For this review, take the finished solid that the model builds, in its own axes (mm). Face numbers are marked on the shaded views. A direction names the side the tool comes from. Round coordinates to 2 decimals unless told otherwise and drop trailing zeros. Write each loop counter-clockwise with the first axis right and the second up, starting at its lowest first coordinate (ties: lowest second). Pieces come first, ordered by that corner, then holes. Notation, with made-up numbers: (48, 11) -> (78, 11) arc R8 cw to (78, 24) -> close; hole circle Ø10 at (72, 12.5). An arc over 180 degrees is marked (long way). Answer as CSV lines item,"result". Start each with the question number.
Item 1: Take a section at A-A on y = 11.7. Count the separate pieces of the cut face and the enclosed holes in it, then the cut area to 3 significant figures.
Item 2: Machinability: for the marked faces 1, 2 and 3, which of the approach directions +Z, -Z, +X, -X, +Y, -Y give a long, thin tool a straight path to every point of the face, cutting with its end or side? Answer none if there is none.
Item 3: Wall thickness on probe 1 along X at (y, z) = (11, 8); probe 2 along Z at (x, y) = (13.5, 3.5); probe 3 along Y at (x, z) = (8.75, 7): over which ranges is each line inside the solid? List them lowest first. Write a range as from..to.
Item 4: Take a section at D-D on y = 7.25. Give the boundary of the cut face in (x, z).
Item 5: Take a section at B-B on z = 23.5. Give the boundary of the cut face in (x, y).
Item 6: For pin 1 Ø6.5 at (x, z) = (5.5, 25.5) entering from +Y; pin 2 Ø6 at (x, y) = (9, 13) entering from +Z; pin 3 Ø3.5 at (y, z) = (13, 15.5) entering from -X, all flat-tipped, find the tip position at first contact; note any pin that passes through.
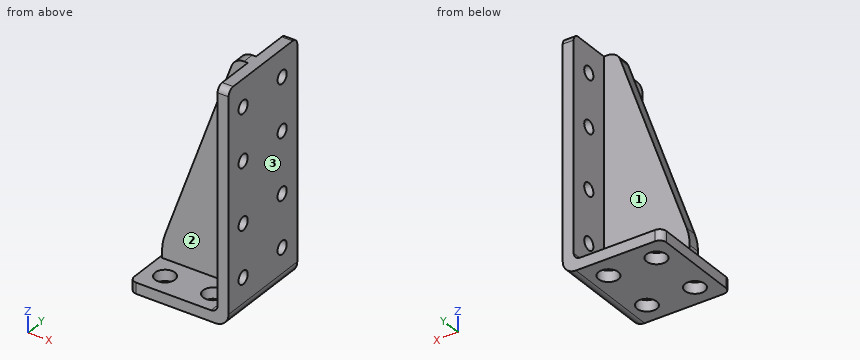
```python
from build123d import *

# Parameters (mm, degrees)
F0_W           = 15
F0_H           = 15
F1_DEPTH       = 1.66
F2_W           = 1.66
F2_H           = 15
F3_DEPTH       = 33.33
F5_DEPTH       = 13
F6_SIZE2       = 31
F6_SIZE        = 11
F7_R           = 1
F8_R           = 2
F9_R           = 8
F10_R          = 1.5
F11_DEPTH      = 25
F12_R          = 1
F13_DEPTH      = 25
F13_DEPTH_BACK = 25


with BuildPart() as f1:
    # F0 (on Top) → F1 (new body)
    with BuildSketch(Plane.XY):
        with Locations((7.5, 7.5)):
            Rectangle(F0_W, F0_H)
    extrude(amount=F1_DEPTH)

    # F2 (on face) → F3 (join)
    with BuildSketch(Plane.XY.offset(1.66)):
        with Locations((14.17, 7.5)):
            Rectangle(F2_W, F2_H)
    extrude(amount=F3_DEPTH)

    # F4 (on face) → F5 (join)
    with BuildSketch(Plane(origin=(13.34, 0, 0), x_dir=(0, -1, 0), z_dir=(-1, 0, 0))):
        Polygon((-6.6, 34.99), (-7.5, 34.99), (-8.4, 34.99), (-8.4, 1.66), (-7.5, 1.66), (-6.6, 1.66), align=None)
    extrude(amount=F5_DEPTH)

    # F6
    f6_edges = [f1.edges().sort_by_distance(p)[0] for p in [
        (0.34, 7.5, 34.99),
    ]]
    f6_side = f1.faces().sort_by_distance((10.61882, 7.5, 34.99))[0]
    chamfer(f6_edges, length=F6_SIZE, length2=F6_SIZE2, reference=f6_side)

    # F7
    f7_edges = [f1.edges().sort_by_distance(p)[0] for p in [
        (0, 0, 0.83),
        (0, 15, 0.83),
        (13.34, 3.3, 1.66),
        (13.34, 11.7, 1.66),
        (14.17, 15, 34.99),
        (14.17, 0, 34.99),
    ]]
    fillet(f7_edges, radius=F7_R)

    # F8
    f8_edges = [f1.edges().sort_by_distance(p)[0] for p in [
        (11.34, 7.5, 34.99),
        (15, 7.5, 0),
    ]]
    fillet(f8_edges, radius=F8_R)

    # F9
    f9_edges = [f1.edges().sort_by_distance(p)[0] for p in [
        (0.34, 7.5, 3.99),
    ]]
    fillet(f9_edges, radius=F9_R)

    # F10 (on face) → F11 (cut)
    with BuildSketch(Plane.XY.offset(1.66)):
        with Locations((3.0819363892, 11.7)):
            Circle(F10_R)
        with Locations((10.3592835367, 11.7)):
            Circle(F10_R)
        with Locations((3.0819363892, 3.3)):
            Circle(F10_R)
        with Locations((10.3592835367, 3.3)):
            Circle(F10_R)
    extrude(amount=-F11_DEPTH, mode=Mode.SUBTRACT)

    # F12 (on face) → F13 (cut, two sides)
    with BuildSketch(Plane(origin=(13.34, 0, 0), x_dir=(0, -1, 0), z_dir=(-1, 0, 0))) as f13_sk:
        with Locations((-11.7, 22.9306016117)):
            Circle(F12_R)
        with Locations((-11.7, 30.8641027659)):
            Circle(F12_R)
        with Locations((-11.7, 13.7193983883)):
            Circle(F12_R)
        with Locations((-11.7, 5.7858972341)):
            Circle(F12_R)
        with Locations((-3.1753151298, 30.8641027659)):
            Circle(F12_R)
        with Locations((-3.1753151298, 22.9306016117)):
            Circle(F12_R)
        with Locations((-3.1753151298, 13.7193983883)):
            Circle(F12_R)
        with Locations((-3.1753151298, 5.7858972341)):
            Circle(F12_R)
    extrude(amount=F13_DEPTH, mode=Mode.SUBTRACT)
    extrude(f13_sk.sketch, amount=-F13_DEPTH_BACK, mode=Mode.SUBTRACT)


solid = f1.part
```
Output values:
1,separate pieces,"7"
1,enclosed holes,"0"
1,area,"56.3 mm^2"
2,face 1,"+Z, -X, +Y"
2,face 2,"+Z, -X, -Y"
2,face 3,"+Z, -Z, +X, +Y, -Y"
3,probe 1,"x = 13.34..15"
3,probe 2,"z = 0.06..4.84, 6.73..12.77, 14.67..21.98, 23.88..29.92, 31.81..34.99"
3,probe 3,"y = 6.6..8.4"
4,outline,"(0, 0) -> (13, 0) arc R2 ccw to (15, 2) -> (15, 34.99) -> (12.75, 34.99) arc R2 ccw to (10.87, 33.66) -> (0.8, 5.29) arc R8 ccw to (0.34, 2.61) -> (0.34, 1.66) -> (0, 1.66) -> close"
5,outline,"(7.26, 6.6) -> (13.34, 6.6) -> (13.34, 4) -> (15, 4) -> (15, 10.88) -> (13.34, 10.88) -> (13.34, 8.4) -> (7.26, 8.4) -> close; (13.34, 0) -> (15, 0) -> (15, 2.35) -> (13.34, 2.35) -> close; (13.34, 12.52) -> (15, 12.52) -> (15, 15) -> (13.34, 15) -> close"
6,pin 1,"stops at y = 8.4"
6,pin 2,"stops at z = 1.66"
6,pin 3,"stops at x = 13.34"
